from build123d import *

# Parameters (mm, degrees)
SKETCH2_W  = 6.858
SKETCH2_H  = 1.2192
SLOT_DEPTH = 1.27


with BuildPart() as part:
    # BodySke → Base-Revolve (revolve)
    with BuildSketch(Plane.XY, mode=Mode.PRIVATE) as base_revolve_sk:
        with BuildLine():
            Line((2.4638, 1.7526), (2.4638, 3.429))
            Line((2.4638, 3.429), (1.1684, 3.429))
            ThreePointArc((1.1684, 3.429), (0.342216437, 3.086783563), (0, 2.2606))
            Line((0, 2.2606), (0, 0))
            Line((0, 0), (53.2638, 0))
            Line((53.2638, 0), (53.2638, 1.7526))
            Line((53.2638, 1.7526), (2.4638, 1.7526))
        make_face()
    revolve(base_revolve_sk.sketch.rotate(Axis((-25.4, 0, 0), (1, 0, 0)), 90), axis=Axis((-25.4, 0, 0), (1, 0, 0)))

    # Sketch2 → Slot (cut)
    with BuildSketch(Plane(origin=(0, 0, 0), x_dir=(0, 0, -1), z_dir=(1, 0, 0))):
        Rectangle(SKETCH2_W, SKETCH2_H)
    extrude(amount=SLOT_DEPTH, mode=Mode.SUBTRACT)


solid = part.part
CAD build for the part. Positions are in the model's coordinates, mm. A direction names the side the tool comes from. Round coordinates to 2 decimals unless told otherwise and drop trailing zeros. Order: outer loops, then holes, each group sorted by start corner. A loop starts at its lowest first (then second) coordinate and runs counter-clockwise, first axis right, second up. Notation, with made-up numbers: M 60,33 L 105,33 A16 ccw 105,45 Z; hole C -13.75,17 d5. An arc over 180 degrees is marked long. Use one line per item in the form item = value.
Q1. Flat gauge pins, fed straight in: P1, Ø1, axis at x = 0.5, z = -1, coming from the +Y side; P2, Ø4, axis at x = 43, y = -0.5, coming from the -Z side; P3, Ø4, axis at x = 47, y = 1, coming from the +Z side. Where does each tip first touch, or does it go through?
Recorded:
P1 = 3.33
P2 = -1.75
P3 = 1.75
Q2. Saw through at C-C on x = 30.5. Give the cut face in (y, z), then the cut area to 3 significant figures.
Recorded:
outline = C 0,0 d3.51
area = 9.65 mm^2
Q3. Two-plate mould, pull along Y, no slides. Class faces 4 (the flat face through (1, 0.61, 0)), 5 (the cylindrical face through (27.51, -0.53, 1.67)), 6 (the flat face through (0, -1, 0)): +Y half, -Y half, draft (parallel to the pull), parting line (faces both ways), or undercut.
Recorded:
face_4 = undercut
face_5 = parting line
face_6 = draft
Q4. Which spindle directions (+Z, -Z, +X, -X, +Y, -Y) get a long thin tool onto all of the face, cutting with end or side? Do faces 1 (the cylindrical face through (1.81, -1.03, 3.27)), 2 (the flat face through (1, -0.61, 0)), 3 (the flat face through (2.464, -1, 2)). Say none if no direction does.
Recorded:
face_1 = +X, -X
face_2 = +Z, -Z, -X
face_3 = +X
Q5. Saw through at B-B on z = 0. Give the cut face in (x, y).
Recorded:
outline = M 0,-2.26 A1.17 ccw 1.17,-3.43 L 2.46,-3.43 L 2.46,-1.75 L 53.26,-1.75 L 53.26,1.75 L 2.46,1.75 L 2.46,3.43 L 1.17,3.43 A1.17 ccw 0,2.26 L 0,0.61 L 1.27,0.61 L 1.27,-0.61 L 0,-0.61 Z
Q6. Probe L1, parallel to X at y = 1.25, z = -1.5; L2, parallel to X at y = 0, z = 0; L3, parallel to Z at x = 18, y = 0.75. List the from-to ranges inside material, lowest first.
Recorded:
L1 = 0 to 2.46
L2 = 1.27 to 53.26
L3 = -1.58 to 1.58
Q7. Saw through at A-A on y = 0. Give the cut face in (x, z).
Recorded:
outline = M 1.27,-3.43 L 2.46,-3.43 L 2.46,-1.75 L 53.26,-1.75 L 53.26,1.75 L 2.46,1.75 L 2.46,3.43 L 1.27,3.43 Z
